Geometry check sheet. Reference: the model listing, model coordinates, mm. A direction names the side the tool comes from. Round coordinates to 2 decimals unless told otherwise and drop trailing zeros. Order: outer loops, then holes, each group sorted by start corner. A loop starts at its lowest first (then second) coordinate and runs counter-clockwise, first axis right, second up.
(1) Material ranges on line 1 along Y through (x, z) = (-9, 48); line 2 along Y through (x, z) = (-49, 47); line 3 along Y through (x, z) = (-29, 47.7), recorded low to high.
(2) Sectioned sample at C-C (x = -9). Record the boundary of the cut face in (y, z), plus the area to 3 significant figures.
(3) Sectioned sample at B-B (x = -41.5). Record the boundary of the cut face in (y, z).
(4) Sectioned sample at D-D (z = 43). Record the boundary of the cut face in (x, y).
(5) Go/stop test with flat-tipped pins: pin 1 (3 mm diameter, centred on x = -10.5, y = 18.5, fed in from -Z); pin 2 (2.5 mm diameter, centred on x = -49, y = 28.3, fed in from +Z). Record where each tip stops, or that it passes through.
(6) Set-up check for faces 1 (the face through (-9, 6.65, 46)), 2 (the face through (-3.503, 16.775, 22.185)), 3 (the face through (-50.11, 29.31, 46.06)): record each of +Z, -Z, +X, -X, +Y, -Y from which the full face is reachable in a straight line by a thin tool's end or side.
(7) Release check for a two-part mould opening along Y. For faces 4 (the face through (-28, 17, 50)), 5 (the face through (-27, 29, 22)) record: +Y half, -Y half, draft (parallel to the pull), parting line (faces both ways), or undercut.
(8) Sectioned sample at A-A (z = 37). Record the boundary of the cut face in (x, y), plus the area to 3 significant figures.
from build123d import *

# Parameters (mm, degrees)
ESQUISSE1_W             = 55
ESQUISSE1_H             = 33
BOSS_EXTRU_1_DEPTH      = 50
ENL_V_MAT_EXTRU_2_DEPTH = 45
CONG_1_R                = 5
ESQUISSE3_R             = 1.5
ENL_V_MAT_EXTRU_3_DEPTH = 10
ENL_V_MAT_EXTRU_4_DEPTH = 2
ESQUISSE5_R             = 1.5
ENL_V_MAT_EXTRU_5_DEPTH = 4
ESQUISSE6_R             = 1.5
ENL_V_MAT_EXTRU_7_DEPTH = 4


with BuildPart() as part:
    # Esquisse1 → Boss.-Extru.1 (new body)
    with BuildSketch(Plane.XY):
        with Locations((-27.5, 16.5)):
            Rectangle(ESQUISSE1_W, ESQUISSE1_H)
    extrude(amount=BOSS_EXTRU_1_DEPTH)

    # Esquisse2 → Enlèv. mat.-Extru.2 (cut)
    with BuildSketch(Plane.XY):
        with BuildLine():
            Line((-38, 29), (-16, 29))
            ThreePointArc((-16, 29), (-3.5, 16.5), (-16, 4))
            Line((-16, 4), (-38, 4))
            ThreePointArc((-38, 4), (-50.5, 16.5), (-38, 29))
        make_face()
    extrude(amount=ENL_V_MAT_EXTRU_2_DEPTH, mode=Mode.SUBTRACT)

    # Congé1
    cong_1_edges = [part.edges().sort_by_distance(p)[0] for p in [
        (0, 0, 25),
        (-55, 0, 25),
        (-55, 33, 25),
        (0, 33, 25),
    ]]
    fillet(cong_1_edges, radius=CONG_1_R)

    # Esquisse3 → Enlèv. mat.-Extru.3 (cut)
    with BuildSketch(Plane.XY.offset(50)):
        with Locations((-29, 9.3)):
            Circle(ESQUISSE3_R)
        with Locations((-9, 19.5)):
            Circle(ESQUISSE3_R)
        with Locations((-9, 9.5)):
            Circle(ESQUISSE3_R)
    extrude(amount=-ENL_V_MAT_EXTRU_3_DEPTH, mode=Mode.SUBTRACT)

    # Esquisse4 → Enlèv. mat.-Extru.4 (cut)
    with BuildSketch(Plane(origin=(0, 0, 45), x_dir=(-1, 0, 0), z_dir=(0, 0, -1))):
        Polygon((27.354551733, 6.45), (30.645448267, 6.45), (32.290896534, 9.3), (30.645448267, 12.15), (27.354551733, 12.15), (25.709103466, 9.3), align=None)
        Polygon((7.354551733, 6.65), (10.645448267, 6.65), (12.290896534, 9.5), (10.645448267, 12.35), (7.354551733, 12.35), (5.709103466, 9.5), align=None)
        Polygon((7.354551733, 16.65), (10.645448267, 16.65), (12.290896534, 19.5), (10.645448267, 22.35), (7.354551733, 22.35), (5.709103466, 19.5), align=None)
    extrude(amount=-ENL_V_MAT_EXTRU_4_DEPTH, mode=Mode.SUBTRACT)

    # Esquisse5 → Enlèv. mat.-Extru.5 (cut)
    with BuildSketch(Plane.XY.offset(50)):
        with Locations((-49, 28.3)):
            Circle(ESQUISSE5_R)
        with Locations((-49, 8.3)):
            Circle(ESQUISSE5_R)
    extrude(amount=-ENL_V_MAT_EXTRU_5_DEPTH, mode=Mode.SUBTRACT)

    # Esquisse6 → Enlèv. mat.-Extru.7 (cut)
    with BuildSketch(Plane.XY.offset(46)):
        with Locations((-49, 28.3)):
            Circle(ESQUISSE6_R)
        with Locations((-49, 8.3)):
            Circle(ESQUISSE6_R)
    extrude(amount=-ENL_V_MAT_EXTRU_7_DEPTH, mode=Mode.SUBTRACT)


solid = part.part
Answer below:
1. line 1: y = 0 to 8, 11 to 18, 21 to 33
1. line 2: y = 0 to 6.8, 9.8 to 26.8, 29.8 to 33
1. line 3: y = 0 to 7.8, 10.8 to 33
2. outline: (0, 0) - (6.14, 0) - (6.14, 45) - (6.65, 45) - (6.65, 47) - (8, 47) - (8, 50) - (0, 50) - close; (11, 47) - (12.35, 47) - (12.35, 45) - (16.65, 45) - (16.65, 47) - (18, 47) - (18, 50) - (11, 50) - close; (21, 47) - (22.35, 47) - (22.35, 45) - (26.86, 45) - (26.86, 0) - (33, 0) - (33, 50) - (21, 50) - close
2. area: 677 mm2
3. outline: (0, 0) - (4.5, 0) - (4.5, 45) - (28.5, 45) - (28.5, 0) - (33, 0) - (33, 50) - (0, 50) - close
4. outline: (-55, 5) arc R5 ccw to (-50, 0) - (-5, 0) arc R5 ccw to (0, 5) - (0, 28) arc R5 ccw to (-5, 33) - (-50, 33) arc R5 ccw to (-55, 28) - close; hole circle Ø3 at (-49, 28.3); hole (-48.5, 9.71) arc R1.5 ccw (long way) to (-47.5, 8.38) arc R12.5 ccw to (-38, 4) - (-16, 4) arc R12.5 ccw to (-16, 29) - (-38, 29) arc R12.5 ccw to start
5. pin 1: stops at z = 45
5. pin 2: stops at z = 42
6. face 1: none
6. face 2: -Z
6. face 3: +Z
7. face 4: draft
7. face 5: undercut
8. outline: (-55, 5) arc R5 ccw to (-50, 0) - (-5, 0) arc R5 ccw to (0, 5) - (0, 28) arc R5 ccw to (-5, 33) - (-50, 33) arc R5 ccw to (-55, 28) - close; hole (-38, 4) - (-16, 4) arc R12.5 ccw to (-16, 29) - (-38, 29) arc R12.5 ccw to start
8. area: 753 mm2
